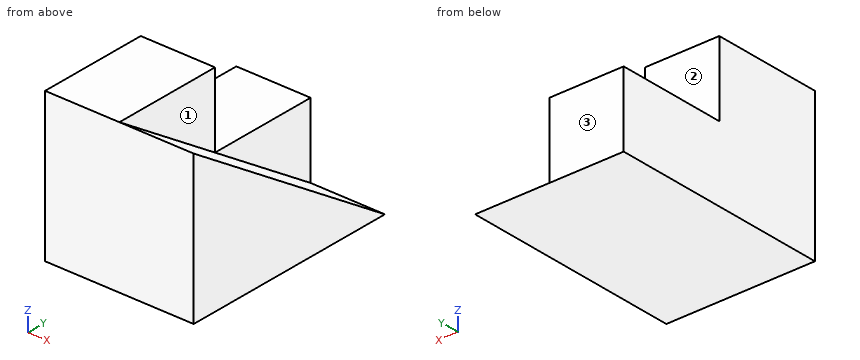
```python
from build123d import *

# Parameters (mm, degrees)
F2_DEPTH = 25.4
F3_DEPTH = 12.7


with BuildPart() as f2:
    # F0 (on Right) → F2 (new body)
    with BuildSketch(Plane.YZ):
        Polygon((0, 0), (-38.1, 25.4), (-38.1, 0), align=None)
    extrude(amount=F2_DEPTH)

    # F1 (on Right) → F3 (join)
    with BuildSketch(Plane.YZ):
        Polygon((-19.05, 25.4), (-38.1, 25.4), (-19.05, 12.7), align=None)
        Polygon((0, 12.7), (-19.05, 12.7), (0, 0), align=None)
    extrude(amount=F3_DEPTH)


solid = f2.part
```
CAD build for the part. Positions are in the model's coordinates, mm. Face numbers are marked on the shaded views. A direction names the side the tool comes from. Round coordinates to 2 decimals unless told otherwise and drop trailing zeros. Write each loop counter-clockwise with the first axis right and the second up, starting at its lowest first coordinate (ties: lowest second). Pieces come first, ordered by that corner, then holes.
Item 1: Band-saw the part on C-C on x = 14.75. Write the cut outline in (y, z).
Filled in:
outline: (-38.1, 0) - (0, 0) - (-38.1, 25.4) - close
Item 2: Band-saw the part on A-A on z = 18. Write the cut outline in (x, y).
Filled in:
outline: (0, -38.1) - (25.4, -38.1) - (25.4, -27) - (12.7, -27) - (12.7, -19.05) - (0, -19.05) - close
Item 3: Drill centre lines: L1, parallel to X at y = -5, z = 9.75; L2, parallel to Y at x = 3.25, z = 22.5. Where is each one in solid material? Low to high.
Filled in:
L1: x = 0 to 12.7
L2: y = -38.1 to -19.05
Item 4: Drop flat-ended pins along their axis: pin 1 Ø4 at (x, z) = (9.5, 17.5) entering from +Y; pin 2 Ø3 at (x, y) = (15, -22.5) entering from +Z; pin 3 Ø10 at (y, z) = (-8.5, 21.5) entering from -X; pin 4 Ø10 at (x, y) = (3.5, -9) entering from +Z. Give the stop position or say it passes through.
Filled in:
pin 1: stops at y = -19.05
pin 2: stops at z = 16
pin 3: passes through
pin 4: stops at z = 12.7
Item 5: Tool access for the marked faces 1, 2 and 3: list every direction of +Z, -Z, +X, -X, +Y, -Y with a clear straight run to the whole face (end or side of a thin tool).
Filled in:
face 1: +Z, +X, +Y
face 2: +Z, +X, -X, +Y
face 3: +Z, -Z, +X, -X, +Y
Item 6: Band-saw the part on B-B on y = -24. Write the cut outline in (x, z).
Filled in:
outline: (0, 0) - (25.4, 0) - (25.4, 16) - (12.7, 16) - (12.7, 25.4) - (0, 25.4) - close
